The figure shows three views and two pictorial views of one solid part (mm, origin at its lowest corner). Answer the questions. A direction names the side the tool comes from. Coordinates: 2 decimals unless noted, no trailing zeros. Order: outer loops, then holes, each group sorted by start corner. A loop starts at its lowest first (then second) coordinate and runs counter-clockwise, first axis right, second up. Notation, with made-up numbers: (-15.75, 5.5) -> (13.25, 5.5) arc R18 cw to (13.25, 24.5) -> close; hole circle Ø8 at (-13, 67). An arc over 180 degrees is marked (long way). Return JSON: item names as keys, results as strings.
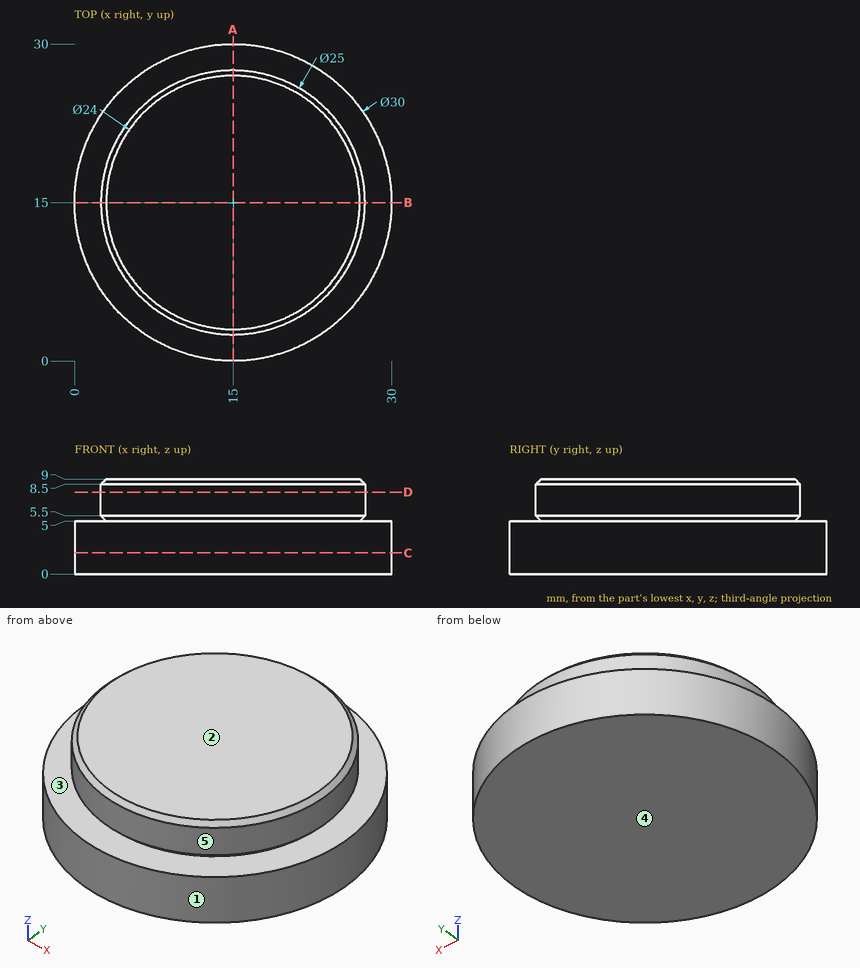
1. Each of these flat-tipped pins is pushed along its axis until it touches: pin 1 Ø3 at (x, y) = (24, 16) entering from -Z; pin 2 Ø2 at (x, y) = (5.5, 24) entering from +Z; pin 3 Ø1 at (x, z) = (26, 2.5) entering from -Y; pin 4 Ø5 at (x, z) = (20.5, 5) entering from -Y. Where does it stop, or does it pass through?
Answer block:
{"pin 1": "stops at z = 0", "pin 2": "stops at z = 8.91", "pin 3": "stops at y = 4.29", "pin 4": "stops at y = 0.3"}
2. The part is cut by section A-A on x = 15. Give the vertices of the cut face in (y, z), and give its area (4 significant figures).
Answer block:
{"outline": "(0, 0) -> (30, 0) -> (30, 5) -> (27, 5) -> (27.5, 5.5) -> (27.5, 8.5) -> (27, 9) -> (3, 9) -> (2.5, 8.5) -> (2.5, 5.5) -> (3, 5) -> (0, 5) -> close", "area": "249.5 mm2"}
3. Determine the mould class of the marked faces 1, 2 and 3 for opening direction Z: pulls with the +Z half, pulls with the -Z half, needs draft (parallel to the pull), parting line crosses it, or undercut.
Answer block:
{"face 1": "needs draft", "face 2": "pulls with the +Z half", "face 3": "undercut"}
4. Consider line 1 (Z direction, x = 1.5, y = 11.25); line 2 (Y direction, x = 18.75, z = 5.25); line 3 (Y direction, x = 13, z = 4.25). Determine where each line is inside the solid, lowest interval first. Write a range as from..to.
Answer block:
{"line 1": "z = 0..5", "line 2": "y = 3.34..26.66", "line 3": "y = 0.13..29.87"}
5. The part is cut by section C-C on z = 2. Give the vertices of the cut face in (x, y), and give its area (3 significant figures).
Answer block:
{"outline": "circle Ø30 at (15, 15)", "area": "707 mm2"}
6. For the marked faces 4 and 5, determine the directions among +Z, -Z, +X, -X, +Y, -Y from which every point of the face is accessible in a straight line to the end or side of a thin tool.
Answer block:
{"face 4": "-Z, +X, -X, +Y, -Y", "face 5": "+Z"}
7. The part is cut by section D-D on z = 7.75. Give the vertices of the cut face in (x, y).
Answer block:
{"outline": "circle Ø25 at (15, 15)"}
